Check sheet for the modelled part. Datum: model origin and axes. Units: mm. Face numbers are marked on the shaded views. A direction names the side the tool comes from. Give positions to 0.01 mm unless a question says otherwise; leave off trailing zeros. Order: outer loops, then holes, each group sorted by start corner. A loop starts at its lowest first (then second) coordinate and runs counter-clockwise, first axis right, second up.
Item 1: Sectioned sample at C-C on z = 10. Record the boundary of the cut face in (x, y), and give its area (3 significant figures).
Item 2: Material ranges on line 1 along Z through (x, y) = (5.5, -8.5); line 2 along Z through (x, y) = (-3, -9); line 3 along X through (y, z) = (-1, 10), recorded low to high.
Item 3: Sectioned sample at B-B on z = 5. Record the boundary of the cut face in (x, y).
Item 4: Gauge pin test, flat ends, axial feed: P1, Ø1.5, axis at y = -8, z = 1.5, coming from the -X side; P2, Ø6, axis at x = 1, y = -7, coming from the +Z side; P3, Ø5, axis at x = -3.5, z = 3.5, coming from the -Y side. Record the tip position at first contact, or that the pin passes through.
Item 5: Access from +Z, -Z, +X, -X, +Y, -Y to the whole of each face (thin tool, end or side, straight path). Record for the marked faces 1 and 2.
from build123d import *

# Parameters (mm, degrees)
F0_R      = 11
F1_DEPTH  = 3
F5_R      = 5.5
F6_DEPTH  = 1
F7_R      = 4
F8_DEPTH  = 4
F9_R      = 2.85
F10_DEPTH = 3
F11_R     = 0.29999


# Not quite as in the source:
# - a fillet or chamfer is up to 0.001 mm smaller than in the source, because OpenCascade refuses the exact size


with BuildPart() as f1:
    # F0 (on Top) → F1 (new body)
    with BuildSketch(Plane.XY):
        Circle(F0_R)
    extrude(amount=F1_DEPTH)

    # F3 (on Front) → F4 (revolve, cut)
    with BuildSketch(Plane.XZ):
        with BuildLine():
            Line((0, -42.4037037037), (0, 2.7))
            ThreePointArc((0, 2.7), (-22.5518518519, -19.8518518519), (0, -42.4037037037))
        make_face()
    revolve(axis=Axis((0, 0, -19.8518518519), (0, 0, -1)), mode=Mode.SUBTRACT)

    # F5 (on face) → F6 (join)
    with BuildSketch(Plane.XY.offset(3)):
        Circle(F5_R)
    extrude(amount=F6_DEPTH)

    # F7 (on face) → F8 (join)
    with BuildSketch(Plane.XY.offset(4)):
        Circle(F7_R)
    extrude(amount=F8_DEPTH)

    # F9 (on face) → F10 (join)
    with BuildSketch(Plane.XY.offset(8)):
        Circle(F9_R)
    extrude(amount=F10_DEPTH)

    # F11 (radius 0.3 in the source; OpenCascade refuses exactly that, so slightly less here)
    f11_edges = [f1.edges().sort_by_distance(p)[0] for p in [
        (-11, 0, 0),
    ]]
    fillet(f11_edges, radius=F11_R)


solid = f1.part
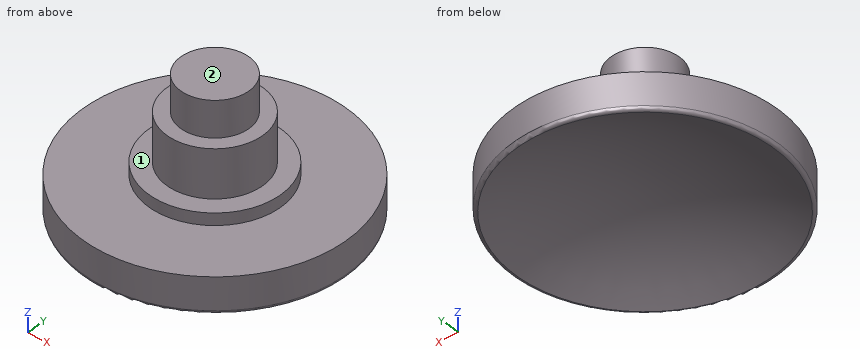
Report:
1. outline: circle Ø5.7 at (0, 0)
1. area: 25.5 mm2
2. line 1: z = 0.3 to 3
2. line 2: z = 0.61 to 3
2. line 3: x = -2.67 to 2.67
3. outline: circle Ø8 at (0, 0)
4. P1: stops at x = -8.27
4. P2: stops at z = 4
4. P3: stops at y = -10.95
5. face 1: +Z
5. face 2: +Z, +X, -X, +Y, -Y
